Geometry check sheet. Reference: the model listing, model coordinates, mm. A direction names the side the tool comes from. Round coordinates to 2 decimals unless told otherwise and drop trailing zeros. Write each loop counter-clockwise with the first axis right and the second up, starting at its lowest first coordinate (ties: lowest second). Pieces come first, ordered by that corner, then holes. Notation, with made-up numbers: (46, -19) -> (78, -19) arc R13 ccw to (78, -2) -> close; hole circle Ø8 at (41, 65). An arc over 180 degrees is marked (long way). Use a Markdown table: item, result.
```python
from build123d import *


with BuildPart() as part:
    # 草图2 → 旋转1 (revolve)
    with BuildSketch(Plane.XY, mode=Mode.PRIVATE) as revolve_1_sk:
        Polygon((5, 2.5), (5, -2.5), (6, -2.5), (6, -2.25), (8.5, -2.25), (8.5, -2.5), (9.5, -2.5), (9.5, 1.5), (10.5, 1.5), (10.5, 2.5), (9.5, 2.5), (8.5, 2.5), (8.5, 2.25), (6, 2.25), (6, 2.5), align=None)
    revolve(revolve_1_sk.sketch.rotate(Axis((0, 0, 0), (0, 1, 0)), 90), axis=Axis((0, 0, 0), (0, 1, 0)))


solid = part.part
```
(1) Gauge pin test, flat ends, axial feed: pin 1 Ø1 at (x, y) = (-6, -2) entering from -Z; pin 2 Ø1 at (x, y) = (-6.5, -1) entering from -Z; pin 3 Ø3 at (x, y) = (-6, -0.5) entering from -Z. Record the tip position at first contact, or that the pin passes through.
A:
| item | result |
|---|---|
| pin 1 | stops at z = -7.75 |
| pin 2 | stops at z = -7.37 |
| pin 3 | stops at z = -8.37 |
(2) Thickness scan on line 1 (X direction, y = -2.4, z = 0); line 2 (X direction, y = 1.25, z = 0); line 3 (Y direction, x = -2.75, z = 7). Record the ranges inside material, lowest first.
A:
| item | result |
|---|---|
| line 1 | x = -9.5 to -8.5, -6 to -5, 5 to 6, 8.5 to 9.5 |
| line 2 | x = -9.5 to -5, 5 to 9.5 |
| line 3 | y = -2.25 to 2.25 |
(3) Section check B-B on x = 0. Record the cut outline in (y, z).
A:
| item | result |
|---|---|
| outline | (-2.5, -9.5) -> (1.5, -9.5) -> (1.5, -10.5) -> (2.5, -10.5) -> (2.5, -8.5) -> (2.25, -8.5) -> (2.25, -6) -> (2.5, -6) -> (2.5, -5) -> (-2.5, -5) -> (-2.5, -6) -> (-2.25, -6) -> (-2.25, -8.5) -> (-2.5, -8.5) -> close; (-2.5, 5) -> (2.5, 5) -> (2.5, 6) -> (2.25, 6) -> (2.25, 8.5) -> (2.5, 8.5) -> (2.5, 10.5) -> (1.5, 10.5) -> (1.5, 9.5) -> (-2.5, 9.5) -> (-2.5, 8.5) -> (-2.25, 8.5) -> (-2.25, 6) -> (-2.5, 6) -> close |
(4) Section check A-A on z = 0. Record the cut outline in (x, y).
A:
| item | result |
|---|---|
| outline | (-10.5, 1.5) -> (-9.5, 1.5) -> (-9.5, -2.5) -> (-8.5, -2.5) -> (-8.5, -2.25) -> (-6, -2.25) -> (-6, -2.5) -> (-5, -2.5) -> (-5, 2.5) -> (-6, 2.5) -> (-6, 2.25) -> (-8.5, 2.25) -> (-8.5, 2.5) -> (-10.5, 2.5) -> close; (5, -2.5) -> (6, -2.5) -> (6, -2.25) -> (8.5, -2.25) -> (8.5, -2.5) -> (9.5, -2.5) -> (9.5, 1.5) -> (10.5, 1.5) -> (10.5, 2.5) -> (8.5, 2.5) -> (8.5, 2.25) -> (6, 2.25) -> (6, 2.5) -> (5, 2.5) -> close |
(5) Section check C-C on y = -0.6. Record the cut outline in (x, z), plus the area to 3 significant figures.
A:
| item | result |
|---|---|
| outline | circle Ø19 at (0, 0); hole circle Ø10 at (0, 0) |
| area | 205 mm2 |
(6) Access from +Z, -Z, +X, -X, +Y, -Y to the whole of each face (thin tool, end or side, straight path). Record for faces 1 (the face through (-6, -2.25, 2)), 2 (the face through (-6, 2.25, -2)), 3 (the face through (-3.2, 2, -10)).
A:
| item | result |
|---|---|
| face 1 | -Y |
| face 2 | +Y |
| face 3 | +Y, -Y |
(7) Release check for a two-part mould opening along Z. For faces 4 (the face through (0, 2.5, -9)), 5 (the face through (9.274, -0.472, 2.059)), 6 (the face through (0, 0, 5)) record: +Z half, -Z half, draft (parallel to the pull), parting line (faces both ways), or undercut.
A:
| item | result |
|---|---|
| face 4 | draft |
| face 5 | parting line |
| face 6 | undercut |
(8) Section check D-D on z = 9. Record the cut outline in (x, y).
A:
| item | result |
|---|---|
| outline | (-5.41, 1.5) -> (-3.04, 1.5) -> (-3.04, -2.5) -> (3.04, -2.5) -> (3.04, 1.5) -> (5.41, 1.5) -> (5.41, 2.5) -> (-5.41, 2.5) -> close |
